Could you check a few things on this model? Use its own coordinates, in mm. Face numbers are marked on the shaded views. A direction names the side the tool comes from. Give positions to 0.01 mm unless a question says otherwise; leave off trailing zeros. Order: outer loops, then holes, each group sorted by start corner. A loop starts at its lowest first (then second) coordinate and runs counter-clockwise, first axis right, second up. Notation, with made-up numbers: (67, -40) -> (89, -40) arc R31 cw to (89, -15) -> close; hole circle Ø9 at (29, 28.5). An arc over 180 degrees is marked (long way). One line per item, written item: value.
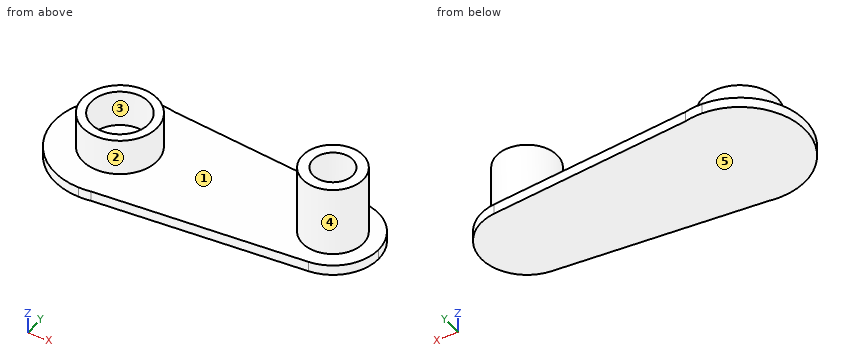
```python
from build123d import *

# Parameters (mm, degrees)
F1_DEPTH = 7
F2_R     = 20.8798
F2_R_2   = 13.684699
F3_DEPTH = 48
F4_R     = 25.632052
F4_R_2   = 19.647778
F5_DEPTH = 25


with BuildPart() as f1:
    # F0 (on Top) → F1 (new body)
    with BuildSketch(Plane.XY):
        with BuildLine():
            Line((-78.980386, 43.715201), (-91.017656, 44.785673))
            ThreePointArc((-91.017656, 44.785673), (-133.756226, -1.040908), (-88.936403, -44.834108))
            Line((-88.936403, -44.834108), (-80.883583, -44.105383))
            ThreePointArc((-80.883583, -44.105383), (-54.502824, -28.715457), (-44.100093, 0))
            ThreePointArc((-44.100093, 0), (-53.888748, 27.962715), (-78.980386, 43.715201))
        make_face()
        with BuildLine():
            ThreePointArc((-78.980386, 43.715201), (-84.962788, 44.657868), (-91.017656, 44.785673))
            Line((-91.017656, 44.785673), (-78.980386, 43.715201))
        make_face()
        with BuildLine():
            Line((-80.883583, -44.105383), (-88.936403, -44.834108))
            ThreePointArc((-88.936403, -44.834108), (-84.893531, -44.651655), (-80.883583, -44.105383))
        make_face()
        with BuildLine():
            Line((60.404596, 31.319727), (-78.980386, 43.715201))
            ThreePointArc((-78.980386, 43.715201), (-53.888748, 27.962715), (-44.100093, 0))
            ThreePointArc((-44.100093, 0), (-54.502824, -28.715457), (-80.883583, -44.105383))
            Line((-80.883583, -44.105383), (60.453168, -31.31537))
            ThreePointArc((60.453168, -31.31537), (26.17602, -0.024383), (60.404596, 31.319727))
        make_face()
        with BuildLine():
            ThreePointArc((89.06267, 0), (80.816977, 21.226225), (60.404596, 31.319727))
            ThreePointArc((60.404596, 31.319727), (26.17602, -0.024383), (60.453168, -31.31537))
            ThreePointArc((60.453168, -31.31537), (80.83343, -21.20823), (89.06267, 0))
        make_face()
    extrude(amount=F1_DEPTH)

    # F2 (on face) → F3 (join)
    with BuildSketch(Plane.XY.offset(7)):
        with Locations((57.61934, 0)):
            Circle(F2_R)
        with Locations((57.61934, 0)):
            Circle(F2_R_2, mode=Mode.SUBTRACT)
    extrude(amount=F3_DEPTH)

    # F4 (on face) → F5 (join)
    with BuildSketch(Plane.XY.offset(7)):
        with Locations((-88.934202, 0)):
            Circle(F4_R)
        with Locations((-88.934202, 0)):
            Circle(F4_R_2, mode=Mode.SUBTRACT)
    extrude(amount=F5_DEPTH)


solid = f1.part
```
1) If I drill on line 1 along Z through (x, y) = (11, -13.5); line 2 along Z through (x, y) = (-99, 22); line 3 along Y through (x, z) = (-88, 15), over which ranges is the centre line in solid material (lowest first)?
Answer below:
line 1: z = 0 to 7
line 2: z = 0 to 32
line 3: y = -25.62 to -19.63, 19.63 to 25.62
2) Suppose I cut it at B-B, the plane y = -7.5. Write out the boundary of the cut face in (x, z), then the cut area to 3 significant figures.
Answer below:
outline: (-133.14, 0) -> (88.16, 0) -> (88.16, 7) -> (77.11, 7) -> (77.11, 55) -> (69.07, 55) -> (69.07, 7) -> (46.17, 7) -> (46.17, 55) -> (38.13, 55) -> (38.13, 7) -> (-64.42, 7) -> (-64.42, 32) -> (-70.77, 32) -> (-70.77, 7) -> (-107.09, 7) -> (-107.09, 32) -> (-113.44, 32) -> (-113.44, 7) -> (-133.14, 7) -> close
area: 2,640 mm2
3) Suppose I cut it at A-A, the plane z = 15. Write out the boundary of the cut face in (x, y).
Answer below:
outline: circle Ø51.26 at (-88.93, 0); circle Ø41.76 at (57.62, 0); hole circle Ø39.3 at (-88.93, 0); hole circle Ø27.37 at (57.62, 0)
4) Suppose I cut it at D-D, the plane y = 5. Write out the boundary of the cut face in (x, z), then the cut area to 3 significant figures.
Answer below:
outline: (-133.49, 0) -> (88.66, 0) -> (88.66, 7) -> (77.89, 7) -> (77.89, 55) -> (70.36, 55) -> (70.36, 7) -> (44.88, 7) -> (44.88, 55) -> (37.35, 55) -> (37.35, 7) -> (-63.79, 7) -> (-63.79, 32) -> (-69.93, 32) -> (-69.93, 7) -> (-107.94, 7) -> (-107.94, 32) -> (-114.07, 32) -> (-114.07, 7) -> (-133.49, 7) -> close
area: 2,590 mm2
5) For the marked faces 4 and 5, which set-ups out of +Z, -Z, +X, -X, +Y, -Y let a thin tool reach every point of the face, with its end or its side?
Answer below:
face 4: +Z
face 5: -Z, +X, -X, +Y, -Y
6) We'd pull the mould along Y, two halves only. Please class the marked faces 1, 2 and 3: +Y half, -Y half, draft (parallel to the pull), parting line (faces both ways), or undercut.
Answer below:
face 1: draft
face 2: parting line
face 3: undercut
7) For P1, Ø8, axis at x = 58.5, y = 2, coming from the +Z side; P2, Ø3, axis at y = 22.5, z = 43.5, coming from the +X side; P3, Ø12, axis at y = 9.5, z = 28.5, coming from the +X side; P4, Ø10, axis at x = -71.5, y = 12.5, coming from the +Z side, each with a flat end and sliding along its axis, tell me the tip position at first contact or that it passes through.
Answer below:
P1: stops at z = 7
P2: passes through
P3: stops at x = 78.2
P4: stops at z = 32
8) Suppose I cut it at C-C, the plane x = -37. Write out the boundary of the cut face in (y, z).
Answer below:
outline: (-40.13, 0) -> (39.98, 0) -> (39.98, 7) -> (-40.13, 7) -> close
